from build123d import *

# Parameters (mm, degrees)
CYLINDER008_R                    = 6.3
CYLINDER008_DEPTH                = 50
CYLINDER009_R                    = 9.5
CYLINDER009_DEPTH                = 13
CYLINDER007_R                    = 9.5
CYLINDER007_DEPTH                = 20
CYLINDER006_R                    = 7
CYLINDER006_DEPTH                = 30
LINEAREXTRUDE002_DEPTH           = 8
LINEAREXTRUDE003_DEPTH           = 8
LINEAREXTRUDE003_PLACEMENT_ANGLE = 34
CYLINDER005_R                    = 11
CYLINDER005_DEPTH                = 25
CYLINDER003_R                    = 6.3
CYLINDER003_DEPTH                = 50
CYLINDER004_R                    = 9.5
CYLINDER004_DEPTH                = 13
CYLINDER002_R                    = 9.5
CYLINDER002_DEPTH                = 20
CYLINDER001_R                    = 7
CYLINDER001_DEPTH                = 30
LINEAREXTRUDE_DEPTH              = 8
LINEAREXTRUDE001_DEPTH           = 8
LINEAREXTRUDE001_PLACEMENT_ANGLE = 34
CYLINDER_R                       = 11
CYLINDER_DEPTH                   = 25


with BuildPart() as cylinder008:
    # cylinder008 → cylinder008 (new body)
    with BuildSketch(Plane.XY.offset(-15)):
        Circle(CYLINDER008_R)
    extrude(amount=CYLINDER008_DEPTH)


with BuildPart() as cylinder009:
    # cylinder009 → cylinder009 (new body)
    with BuildSketch(Plane.XY.offset(13.5)):
        Circle(CYLINDER009_R)
    extrude(amount=CYLINDER009_DEPTH)


with BuildPart() as group003:
    # cylinder007 → cylinder007 (new body)
    with BuildSketch(Plane.XY.offset(-30)):
        Circle(CYLINDER007_R)
    extrude(amount=CYLINDER007_DEPTH)

    # Group003: union cylinder008, cylinder009
    add(cylinder008.part)
    add(cylinder009.part)


with BuildPart() as cylinder006:
    # cylinder006 → cylinder006 (new body)
    with BuildSketch(Plane.XY.offset(-15)):
        Circle(CYLINDER006_R)
    extrude(amount=CYLINDER006_DEPTH)


with BuildPart() as linearextrude002:
    # RefineLinearExtrude002 → LinearExtrude002 (new body)
    with BuildSketch(Plane(origin=(0, 0, 0), x_dir=(0, -1, 0), z_dir=(0, 0, -1))):
        Polygon((-12.124356, -7), (0, -14), (12.124356, -7), (12.124356, 7), (0, 14), (-12.124356, 7), align=None)
    extrude(amount=-LINEAREXTRUDE002_DEPTH)


with BuildPart() as linearextrude002_1:
    # LinearExtrude002 placement: moved
    add(linearextrude002.part.moved(Location((0, 0, -4))))


with BuildPart() as linearextrude003:
    # RefineLinearExtrude003 → LinearExtrude003 (new body)
    with BuildSketch(Plane(origin=(0, 0, 0), x_dir=(0, -1, 0), z_dir=(0, 0, -1))):
        Polygon((-12.124356, -7), (0, -14), (12.124356, -7), (12.124356, 7), (0, 14), (-12.124356, 7), align=None)
    extrude(amount=-LINEAREXTRUDE003_DEPTH)


with BuildPart() as linearextrude003_1:
    # LinearExtrude003 placement: moved
    add(linearextrude003.part.moved(Location((0, 0, 11))).rotate(Axis((0, 0, 11), (0, 0, 1)), LINEAREXTRUDE003_PLACEMENT_ANGLE))


with BuildPart() as difference001:
    # cylinder005 → cylinder005 (new body)
    with BuildSketch(Plane.XY.offset(-22.5)):
        Circle(CYLINDER005_R)
    extrude(amount=CYLINDER005_DEPTH)

    # Group002: union cylinder006, LinearExtrude002, LinearExtrude003
    add(cylinder006.part)
    add(linearextrude002_1.part)
    add(linearextrude003_1.part)

    # difference001: cut Group003
    add(group003.part, mode=Mode.SUBTRACT)


with BuildPart() as cylinder003:
    # cylinder003 → cylinder003 (new body)
    with BuildSketch(Plane.XY.offset(-15)):
        Circle(CYLINDER003_R)
    extrude(amount=CYLINDER003_DEPTH)


with BuildPart() as cylinder004:
    # cylinder004 → cylinder004 (new body)
    with BuildSketch(Plane.XY.offset(13.5)):
        Circle(CYLINDER004_R)
    extrude(amount=CYLINDER004_DEPTH)


with BuildPart() as group001:
    # cylinder002 → cylinder002 (new body)
    with BuildSketch(Plane.XY.offset(-30)):
        Circle(CYLINDER002_R)
    extrude(amount=CYLINDER002_DEPTH)

    # Group001: union cylinder003, cylinder004
    add(cylinder003.part)
    add(cylinder004.part)


with BuildPart() as cylinder001:
    # cylinder001 → cylinder001 (new body)
    with BuildSketch(Plane.XY.offset(-15)):
        Circle(CYLINDER001_R)
    extrude(amount=CYLINDER001_DEPTH)


with BuildPart() as linearextrude:
    # RefineLinearExtrude → LinearExtrude (new body)
    with BuildSketch(Plane(origin=(0, 0, 0), x_dir=(0, -1, 0), z_dir=(0, 0, -1))):
        Polygon((-12.124356, -7), (0, -14), (12.124356, -7), (12.124356, 7), (0, 14), (-12.124356, 7), align=None)
    extrude(amount=-LINEAREXTRUDE_DEPTH)


with BuildPart() as linearextrude_1:
    # LinearExtrude placement: moved
    add(linearextrude.part.moved(Location((0, 0, -4))))


with BuildPart() as linearextrude001:
    # RefineLinearExtrude001 → LinearExtrude001 (new body)
    with BuildSketch(Plane(origin=(0, 0, 0), x_dir=(0, -1, 0), z_dir=(0, 0, -1))):
        Polygon((-12.124356, -7), (0, -14), (12.124356, -7), (12.124356, 7), (0, 14), (-12.124356, 7), align=None)
    extrude(amount=-LINEAREXTRUDE001_DEPTH)


with BuildPart() as linearextrude001_1:
    # LinearExtrude001 placement: moved
    add(linearextrude001.part.moved(Location((0, 0, 11))).rotate(Axis((0, 0, 11), (0, 0, 1)), LINEAREXTRUDE001_PLACEMENT_ANGLE))


with BuildPart() as group004:
    # cylinder → cylinder (new body)
    with BuildSketch(Plane.XY.offset(-22.5)):
        Circle(CYLINDER_R)
    extrude(amount=CYLINDER_DEPTH)

    # Group: union cylinder001, LinearExtrude, LinearExtrude001
    add(cylinder001.part)
    add(linearextrude_1.part)
    add(linearextrude001_1.part)

    # difference: cut Group001
    add(group001.part, mode=Mode.SUBTRACT)

    # Group004: union difference001
    add(difference001.part)


solid = group004.part
Input: part model. Units: mm. Frame: model coordinates. A direction names the side the tool comes from. Coordinates: 2 decimals unless noted, no trailing zeros. Loops run counter-clockwise (first coordinate to the right, second up) from the corner with the lowest first, then second, coordinate; pieces in that order, holes last. Notation, with made-up numbers: (81, 1) -> (95, 1) arc R10 cw to (95, 6) -> close; hole circle Ø4 at (-28, -10.5). An arc over 180 degrees is marked (long way). Write item = value, one per line. Start each with the question number.
Item 1: First-contact query: P1, Ø4, axis at x = 2.5, y = 7, coming from the +Z side; P2, Ø3, axis at y = -9.5, z = 2.5, coming from the +X side; P3, Ø4, axis at x = 1, z = -1, coming from the -Y side. Flat tips, straight axial feed; report the tip coordinate or a pass-through.
Item 2: Cut plane C-C, the plane z = -2. Return loops of the section in (x, y).
Item 3: Reachability of faces 4 (the face through (-10.549, 5.977, -0.056)), 5 (the face through (-6.861, 9.997, 14.944)), 6 (the face through (-2.38, -10.74, -13.38)), 7 (the face through (12.09, 0.94, 14.94)), 8 (the face through (10.549, -5.977, -0.056)) from +Z, -Z, +X, -X, +Y, -Y: full face, straight path, thin tool, end or side. Return the list, or none.
Item 4: Cut plane B-B, the plane y = -10.5. Return loops of the section in (x, z) (3 decimals).
Item 5: Cut plane D-D, the plane y = -2.25. Return loops of the section in (x, z), plus the area to 3 significant figures.
Item 6: Cut plane A-A, the plane x = -2. Return loops of the section in (y, z), plus the area to 3 significant figures.
Item 7: Material intervals for line 1 (Y direction, x = 0, z = -16.5); line 2 (Z direction, x = 3.75, y = 6.75); line 3 (Z direction, x = -4.75, y = -11), sorted ascending.
Item 8: Mould query, pull axis Y, two halves, no side actions, for faces 1 (the face through (-5.23, -10.94, 14.94)), 2 (the face through (6.2, -2, 13.5)), 3 (the face through (6, 6, 4)). Classes: pulls with the +Y half, pulls with the -Y half, needs draft (parallel to the pull), parting line crosses it, or undercut.
Ans:
q1.P1 = 13.5
q1.P2 = 9.38
q1.P3 = -12.12
q2.outline = (-14, 0) -> (-7, -12.12) -> (7, -12.12) -> (14, 0) -> (7, 12.12) -> (-7, 12.12) -> close; hole circle Ø12.6 at (0, 0)
q3.face_4 = -Z, -X, +Y
q3.face_5 = +Z, -X, +Y
q3.face_6 = -Z
q3.face_7 = +Z, +X, +Y
q3.face_8 = -Z, +X, -Y
q4.outline = (-7.938, -4) -> (-3.279, -4) -> (-3.279, -22.5) -> (3.279, -22.5) -> (3.279, -4) -> (7.938, -4) -> (7.938, 4) -> (-7.938, 4) -> close; (-6.13, 11) -> (6.115, 11) -> (6.115, 19) -> (-6.13, 19) -> close
q5.outline = (-12.7, -4) -> (-10.77, -4) -> (-10.77, -22.5) -> (-9.23, -22.5) -> (-9.23, -10) -> (-5.88, -10) -> (-5.88, 13.5) -> (-9.23, 13.5) -> (-9.23, 19) -> (-12, 19) -> (-12, 11) -> (-6.63, 11) -> (-6.63, 4) -> (-12.7, 4) -> close; (5.88, -10) -> (9.23, -10) -> (9.23, -22.5) -> (10.77, -22.5) -> (10.77, -4) -> (12.7, -4) -> (12.7, 4) -> (6.63, 4) -> (6.63, 11) -> (12.31, 11) -> (12.31, 19) -> (9.23, 19) -> (9.23, 13.5) -> (5.88, 13.5) -> close
q5.area = 280 mm²
q6.outline = (-12.51, 11) -> (-6.71, 11) -> (-6.71, 4) -> (-12.12, 4) -> (-12.12, -4) -> (-10.82, -4) -> (-10.82, -22.5) -> (-9.29, -22.5) -> (-9.29, -10) -> (-5.97, -10) -> (-5.97, 13.5) -> (-9.29, 13.5) -> (-9.29, 19) -> (-12.51, 19) -> close; (5.97, -10) -> (9.29, -10) -> (9.29, -22.5) -> (10.82, -22.5) -> (10.82, -4) -> (12.12, -4) -> (12.12, 4) -> (6.71, 4) -> (6.71, 11) -> (13.28, 11) -> (13.28, 19) -> (9.29, 19) -> (9.29, 13.5) -> (5.97, 13.5) -> close
q6.area = 279 mm²
q7.line_1 = -11 to -9.5, 9.5 to 11
q7.line_2 = -10 to 4, 11 to 13.5
q7.line_3 = -4 to 4, 11 to 19
q8.face_1 = pulls with the -Y half
q8.face_2 = undercut
q8.face_3 = needs draft
